from build123d import *

# Parameters (mm, degrees)
BOSS_EXTRUDE1_DEPTH = 45
BOSS_EXTRUDE2_DEPTH = 20
SKETCH3_R           = 12.5
CUT_EXTRUDE1_DEPTH  = 20
BOSS_EXTRUDE3_DEPTH = 20
SKETCH5_R           = 32.5
SKETCH5_R_2         = 17.5
BOSS_EXTRUDE4_DEPTH = 25
FILLET1_R           = 10
SKETCH8_R           = 17.5
CUT_EXTRUDE2_DEPTH  = 182.698096488
RIB2_REACH          = 183.698
SKETCH9_WALL_W      = 469.435460986
SKETCH9_WALL_H      = 16


with BuildPart() as part:
    # Sketch1 → Boss-Extrude1 (new, symmetric)
    with BuildSketch(Plane.XY):
        Polygon((0, 0), (95, 0), (95, 20), (11.547005384, 20), (-30.179491924, 92.27241336), (-47.5, 82.27241336), align=None)
    extrude(amount=BOSS_EXTRUDE1_DEPTH, both=True)

    # Sketch2 → Boss-Extrude2 (add)
    with BuildSketch(Plane(origin=(17.320508076, 10, 0), x_dir=(0, 0, -1), z_dir=(0.8660254037844396, 0.4999999999999982, 0))):
        with BuildLine():
            Line((-45, 70), (-45, 95))
            ThreePointArc((-45, 95), (-70, 70), (-45, 45))
            Line((-45, 45), (-45, 70))
        make_face()
        with BuildLine():
            ThreePointArc((45, 45), (70, 70), (45, 95))
            Line((45, 95), (45, 45))
        make_face()
    extrude(amount=-BOSS_EXTRUDE2_DEPTH)

    # Sketch3 → Cut-Extrude1 (cut)
    with BuildSketch(Plane(origin=(17.320508076, 10, 0), x_dir=(0, 0, -1), z_dir=(0.8660254037844396, 0.4999999999999982, 0))):
        with Locations(Location((-45, 70, 0), (0, 0, 90))):
            Circle(SKETCH3_R)
        with Locations(Location((45, 70, 0), (0, 0, 90))):
            Circle(SKETCH3_R)
    extrude(amount=-CUT_EXTRUDE1_DEPTH, mode=Mode.SUBTRACT)

    # Sketch4 → Boss-Extrude3 (add)
    with BuildSketch(Plane(origin=(0, 20, 0), x_dir=(1, 0, 0), z_dir=(0, 1, 0))):
        with BuildLine():
            Line((95, 45), (95, -45))
            ThreePointArc((95, -45), (140, 0), (95, 45))
        make_face()
    extrude(amount=-BOSS_EXTRUDE3_DEPTH)

    # Sketch5 → Boss-Extrude4 (add)
    with BuildSketch(Plane(origin=(0, 20, 0), x_dir=(1, 0, 0), z_dir=(0, 1, 0))):
        with Locations(Location((95, 0, 0), (0, 0, 180))):
            Circle(SKETCH5_R)
        with Locations(Location((95, 0, 0), (0, 0, 180))):
            Circle(SKETCH5_R_2, mode=Mode.SUBTRACT)
    extrude(amount=BOSS_EXTRUDE4_DEPTH)

    # Fillet1
    fillet1_edges = [part.edges().sort_by_distance(p)[0] for p in [
        (-13.839745962, 43.97114317, 45),
        (-13.839745962, 43.97114317, -45),
    ]]
    fillet(fillet1_edges, radius=FILLET1_R)

    # Sketch8 → Cut-Extrude2 (cut, through all)
    with BuildSketch(Plane(origin=(0, 0, 0), x_dir=(-1, 0, 0), z_dir=(0, -1, 0))):
        with Locations(Location((-95, 0, 0), (0, 0, 90))):
            Circle(SKETCH8_R)
    extrude(amount=-CUT_EXTRUDE2_DEPTH, mode=Mode.SUBTRACT)

    # Sketch9 wall → Rib2 (add, up to next)
    with BuildSketch(Plane(origin=(16.160254038, 68.63620668, 0), x_dir=(0.890812610433, -0.45437087615, 0), z_dir=(0.45437087615, 0.890812610433, 0)), mode=Mode.PRIVATE) as rib2_sk1:
        Rectangle(SKETCH9_WALL_W, SKETCH9_WALL_H)
    rib2_tool1 = extrude(rib2_sk1.sketch, amount=-RIB2_REACH, mode=Mode.PRIVATE) - part.part
    add(rib2_tool1.solids().sort_by_distance((16.160254038, 68.63620668, 0))[0])


solid = part.part
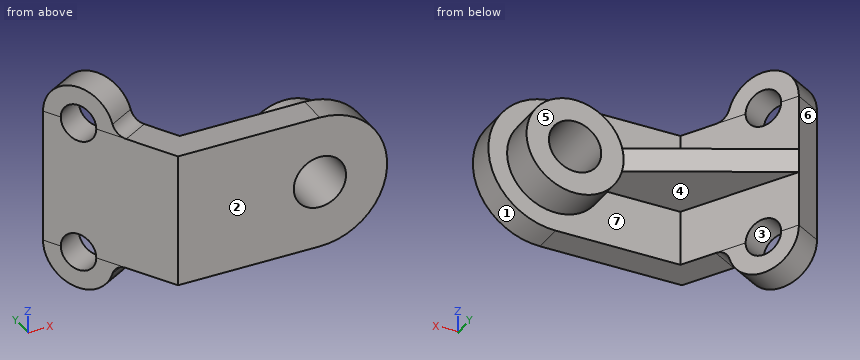
Read the model definition and answer for the solid it produces. Units are mm, in the model's axes. Face numbers are marked on the shaded views. A direction names the side the tool comes from. Coordinates: 2 decimals unless noted, no trailing zeros. Order: outer loops, then holes, each group sorted by start corner. A loop starts at its lowest first (then second) coordinate and runs counter-clockwise, first axis right, second up. Notation, with made-up numbers: (58, 61.25) - (84, 61.25) arc R30 cw to (84, 95.25) - close; hole circle Ø9 at (-24.75, -13.75). An arc over 180 degrees is marked (long way). Use one line per item in the form item = value.
(1) Section A-A, the plane x = 83 is taken. Give the vertices of the cut face in (y, z), then the cut area to 3 significant figures.
Computed values:
outline = (0, -45) - (20, -45) - (20, -30.2) - (45, -30.2) - (45, -12.74) - (0, -12.74) - close; (0, 12.74) - (45, 12.74) - (45, 30.2) - (20, 30.2) - (20, 45) - (0, 45) - close
area = 2,160 mm²
(2) Given pin 1 Ø1 at (x, z) = (113, 5) entering from +Y; pin 2 Ø2 at (y, z) = (25, -8.5) entering from +X; pin 3 Ø2 at (x, y) = (113.5, 12.5) entering from -Z; pin 4 Ø2 at (x, z) = (92, -18.5) entering from -Y, each flat-ended and moving along its own axis, determine where each tip first touches the part or whether it passes through.
Computed values:
pin_1 = 45
pin_2 = 126.62
pin_3 = -41.46
pin_4 = 0
(3) Section D-D, the plane z = -24 is taken. Give the vertices of the cut face in (x, y).
Computed values:
outline = (-47.5, 82.27) - (0, 0) - (133.07, 0) - (133.07, 20) - (116.91, 20) - (116.91, 45) - (73.09, 45) - (73.09, 20) - (11.55, 20) - (-30.18, 92.27) - close
(4) Which of the six approach directions +Z, -Z, +X, -X, +Y, -Y give full straight-line access (tool end or side, diameter ignored) to the marked faces 4, 5, 6 and 7?
Computed values:
face_4 = -Z, +Y
face_5 = +Z, -Z, +X, +Y
face_6 = +Z, -Z, -X, +Y
face_7 = +Y
(5) Section C-C, the plane y = 14.5 is taken. Give the vertices of the cut face in (x, z), then the cut area to 3 significant figures.
Computed values:
outline = (-8.37, -45) - (95, -45) arc R45 ccw to (95, 45) - (-8.37, 45) - close; hole circle Ø35 at (95, 0)
area = 11,500 mm²
(6) Straight lines are drawn through the part: L1, parallel to X at y = 33, z = 11.5; L2, parallel to Y at x = 60.5, z = 42; L3, parallel to Y at x = 114, z = -10. For each, find the intervals that lie inside material, in ascending order.
Computed values:
L1 = -19.05 to 4.04, 64.6 to 81.81, 108.19 to 125.4
L2 = 0 to 20
L3 = 0 to 45
(7) Section B-B, the plane z = -3 is taken. Give the vertices of the cut face in (x, y), then the cut area to 3 significant figures.
Computed values:
outline = (-47.5, 82.27) - (0, 0) - (77.76, 0) - (77.76, 45) - (62.64, 45) - (62.64, 44.93) - (-30.18, 92.27) - close; (112.24, 0) - (139.9, 0) - (139.9, 20) - (127.36, 20) - (127.36, 45) - (112.24, 45) - close
area = 7,540 mm²
(8) For a pull along X with two mould halves and no side action, classify the marked faces 1, 2 and 3 as pulls with the +X half, pulls with the -X half, needs draft (parallel to the pull), parting line crosses it, or undercut.
Computed values:
face_1 = pulls with the +X half
face_2 = needs draft
face_3 = undercut
